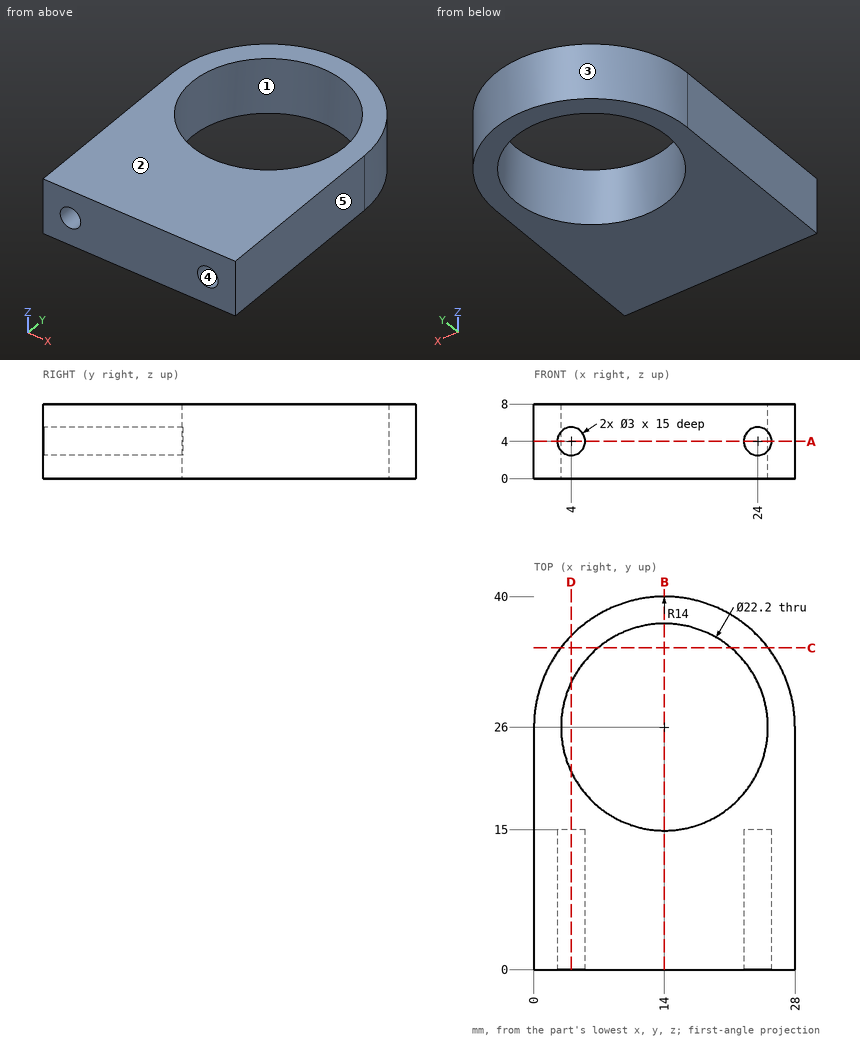
For this review, use the dimensioned drawing (mm, ordinates from the lowest corner) and the shaded views. A direction names the side the tool comes from. Give positions to 0.01 mm unless a question says otherwise; leave off trailing zeros. Order: outer loops, then holes, each group sorted by start corner. A loop starts at its lowest first (then second) coordinate and runs counter-clockwise, first axis right, second up. Notation, with made-up numbers: (64, 72.5) - (98, 72.5) arc R16 ccw to (98, 86.5) - close; hole circle Ø4 at (7.5, 64.25). An arc over 180 degrees is marked (long way). Use a Markdown table: item, result. Add a question column.
(1) Add section A-A on z = 4. Give the boundary of the cut face in (x, y).
(2) Machinability: for the marked faces 4 and 5, which of the approach directions +Z, -Z, +X, -X, +Y, -Y give a long, thin tool a straight path to every point of the face, cutting with its end or side? Answer none if there is none.
(3) Add section C-C on y = 34.5. Give the boundary of the cut face in (x, z).
(4) Add section B-B on x = 14. Give the boundary of the cut face in (y, z).
(5) Mouldability with a two-part tool opening along X and no side actions: class the marked faces 1, 2 and 3 as +X half, -X half, draft (parallel to the pull), parting line (faces both ways), or undercut.
(6) Wall thickness on probe 1 along X at (y, z) = (12.5, 5); probe 2 along Z at (x, y) = (4, 11.75); probe 3 along X at (y, z) = (34, 7.25): over which ranges is each line inside the solid? List them lowest first. Write a range as [from, to].
(7) Clearance check with flat-ended pins moving along their axes: P1, Ø0.9, axis at x = 4.5, z = 4, coming from the -Y side; P2, Ø3, axis at x = 5, z = 4, coming from the +Y side; P3, Ø4, axis at y = 28.5, z = 2.5, coming from the -X side. State where each tip first meets the part, or that it passes through.
(8) Add section D-D on x = 4. Give the boundary of the cut face in (y, z).
Report:
| question | item | result |
|---|---|---|
| 1 | outline | (0, 0) - (2.5, 0) - (2.5, 15) - (5.5, 15) - (5.5, 0) - (22.5, 0) - (22.5, 15) - (25.5, 15) - (25.5, 0) - (28, 0) - (28, 26) arc R14 ccw to (0, 26) - close; hole circle Ø22.2 at (14, 26) |
| 2 | face 4 | -Y |
| 2 | face 5 | +Z, -Z, +X, +Y, -Y |
| 3 | outline | (2.88, 0) - (6.86, 0) - (6.86, 8) - (2.88, 8) - close; (21.14, 0) - (25.12, 0) - (25.12, 8) - (21.14, 8) - close |
| 4 | outline | (0, 0) - (14.9, 0) - (14.9, 8) - (0, 8) - close; (37.1, 0) - (40, 0) - (40, 8) - (37.1, 8) - close |
| 5 | face 1 | undercut |
| 5 | face 2 | draft |
| 5 | face 3 | parting line |
| 6 | probe 1 | x = [0, 2.88], [5.12, 22.88], [25.12, 28] |
| 6 | probe 2 | z = [0, 2.5], [5.5, 8] |
| 6 | probe 3 | x = [2.51, 6.31], [21.69, 25.49] |
| 7 | P1 | stops at y = 15 |
| 7 | P2 | stops at y = 37.82 |
| 7 | P3 | stops at x = 0.01 |
| 8 | outline | (0, 0) - (21.18, 0) - (21.18, 8) - (0, 8) - (0, 5.5) - (15, 5.5) - (15, 2.5) - (0, 2.5) - close; (30.82, 0) - (35.8, 0) - (35.8, 8) - (30.82, 8) - close |
